Geometry: final body of the model. Coordinates: model frame, mm. Face numbers are marked on the shaded views. A direction names the side the tool comes from. Give positions to 0.01 mm unless a question says otherwise; leave off trailing zeros. Order: outer loops, then holes, each group sorted by start corner. A loop starts at its lowest first (then second) coordinate and runs counter-clockwise, first axis right, second up. Notation, with made-up numbers: M 4,8 L 62,8 A20 cw 62,16 Z; hole C 5,82 d10. An arc over 180 degrees is marked long. Use CSV: the item, a comma, the result in double quotes.
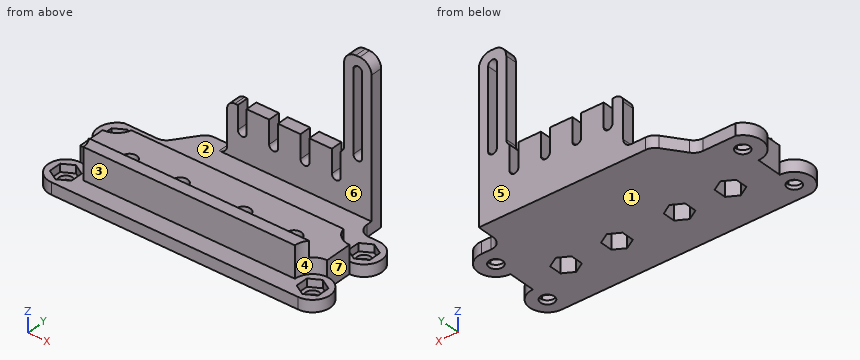
```python
from build123d import *

# Parameters (mm, degrees)
ESQUISSE1_R             = 1.749999998
BOSS_EXTRU_1_DEPTH      = 3
ENL_V_MAT_EXTRU_1_DEPTH = 2
ESQUISSE3_W             = 63
ESQUISSE3_H             = 15
BOSS_EXTRU_2_DEPTH      = 4
ESQUISSE5_W             = 63
ESQUISSE5_H             = 3
BOSS_EXTRU_3_DEPTH      = 4
ESQUISSE4_R             = 4.499999998
ESQUISSE4_R_2           = 4.527692567
ENL_V_MAT_EXTRU_2_DEPTH = 41.723100164
ESQUISSE6_R             = 1.875
ENL_V_MAT_EXTRU_4_DEPTH = 41.538511158
ENL_V_MAT_EXTRU_5_DEPTH = 4
ESQUISSE8_W             = 36.859122618
ESQUISSE8_H             = 3
BOSS_EXTRU_4_DEPTH      = 13
CONG_1_R                = 3
ESQUISSE9_W             = 7
ESQUISSE9_H             = 3
BOSS_EXTRU_5_DEPTH      = 25
CONG_2_R                = 3
CONG_3_R                = 2
CONG_4_R                = 2
ENL_V_MAT_EXTRU_6_DEPTH = 63.211313789


with BuildPart() as part:
    # Esquisse1 → Boss.-Extru.1 (new body)
    with BuildSketch(Plane.XY):
        with BuildLine():
            Line((-33.132757167, 9.120273973), (-23.272060479, 9.120273973))
            Line((-23.272060479, 9.120273973), (-17.824378499, 16.590273973))
            Line((-17.824378499, 16.590273973), (26.292187613, 16.590273973))
            Line((26.292187613, 16.590273973), (26.292187613, 9.120273973))
            Line((26.292187613, 9.120273973), (31.792187613, 9.120273973))
            ThreePointArc((31.792187613, 9.120273973), (36.319880182, 4.592581404), (31.792187613, 0.064888835))
            Line((31.792187613, 0.064888835), (31.792187613, -6.907418596))
            ThreePointArc((31.792187613, -6.907418596), (36.292187613, -11.407418596), (31.792187613, -15.907418596))
            Line((31.792187613, -15.907418596), (-31.207812389, -15.907418596))
            ThreePointArc((-31.207812389, -15.907418596), (-35.707812387, -11.407418595), (-31.207812387, -6.907418596))
            Line((-31.207812387, -6.907418596), (-31.207812387, -0.327318229))
            ThreePointArc((-31.207812387, -0.327318229), (-36.028663215, 3.610334136), (-33.132757167, 9.120273973))
        make_face()
        with Locations((-31.207812387, 4.592581404)):
            Circle(ESQUISSE1_R, mode=Mode.SUBTRACT)
        with Locations((-31.207812387, -11.407418596)):
            Circle(ESQUISSE1_R, mode=Mode.SUBTRACT)
        with Locations((31.792187613, 4.592581404)):
            Circle(ESQUISSE1_R, mode=Mode.SUBTRACT)
        with Locations((31.792187613, -11.407418596)):
            Circle(ESQUISSE1_R, mode=Mode.SUBTRACT)
    extrude(amount=BOSS_EXTRU_1_DEPTH)

    # Esquisse2 → Enlèv. mat.-Extru.1 (cut)
    with BuildSketch(Plane.XY.offset(3)):
        Polygon((-28.457812387, 6.180294644), (-31.207812387, 7.768007885), (-33.957812387, 6.180294644), (-33.957812387, 3.004868164), (-31.207812387, 1.417154924), (-28.457812387, 3.004868164), align=None)
        Polygon((-28.457812387, -9.819705356), (-31.207812387, -8.231992115), (-33.957812387, -9.819705356), (-33.957812387, -12.995131836), (-31.207812387, -14.582845076), (-28.457812387, -12.995131836), align=None)
        Polygon((29.042187613, -9.819705356), (29.042187613, -12.995131836), (31.792187613, -14.582845076), (34.542187613, -12.995131836), (34.542187613, -9.819705356), (31.792187613, -8.231992115), align=None)
        Polygon((29.042187613, 3.004868164), (31.792187613, 1.417154924), (34.542187613, 3.004868164), (34.542187613, 6.180294644), (31.792187613, 7.768007885), (29.042187613, 6.180294644), align=None)
    extrude(amount=-ENL_V_MAT_EXTRU_1_DEPTH, mode=Mode.SUBTRACT)

    # Esquisse3 → Boss.-Extru.2 (add)
    with BuildSketch(Plane.XY.offset(3)):
        with Locations((0.292187613, -3.907418596)):
            Rectangle(ESQUISSE3_W, ESQUISSE3_H)
    extrude(amount=BOSS_EXTRU_2_DEPTH)

    # Esquisse5 → Boss.-Extru.3 (add)
    with BuildSketch(Plane.XY.offset(7)):
        with Locations((0.292187613, -9.907418596)):
            Rectangle(ESQUISSE5_W, ESQUISSE5_H)
    extrude(amount=BOSS_EXTRU_3_DEPTH)

    # Esquisse4 → Enlèv. mat.-Extru.2 (cut, through all)
    with BuildSketch(Plane.XY.offset(3)):
        with Locations((-31.207812387, -11.407418596)):
            Circle(ESQUISSE4_R)
        with Locations((31.792187613, -11.407418596)):
            Circle(ESQUISSE4_R)
        with Locations((-31.207812387, 4.592581404)):
            Circle(ESQUISSE4_R_2)
        with Locations((31.792187613, 4.592581404)):
            Circle(ESQUISSE4_R_2)
    extrude(amount=ENL_V_MAT_EXTRU_2_DEPTH, mode=Mode.SUBTRACT)

    # Esquisse6 → Enlèv. mat.-Extru.4 (cut, through all)
    with BuildSketch(Plane.XY.offset(7)):
        with Locations((-20.707812387, -4.407418596)):
            Circle(ESQUISSE6_R)
        with Locations((-7.707812387, -4.407418596)):
            Circle(ESQUISSE6_R)
    enl_v_mat_extru_4 = extrude(amount=-ENL_V_MAT_EXTRU_4_DEPTH, mode=Mode.SUBTRACT)

    # Esquisse7 → Enlèv. mat.-Extru.5 (cut)
    with BuildSketch(Plane(origin=(0, 0, 0), x_dir=(-1, 0, 0), z_dir=(0, 0, -1))):
        Polygon((23.457812387, -2.819705356), (20.707812387, -1.231992115), (17.957812387, -2.819705356), (17.957812387, -5.995131836), (20.707812387, -7.582845076), (23.457812387, -5.995131836), align=None)
        Polygon((10.457812387, -2.819705356), (7.707812387, -1.231992115), (4.957812387, -2.819705356), (4.957812387, -5.995131836), (7.707812387, -7.582845076), (10.457812387, -5.995131836), align=None)
    enl_v_mat_extru_5 = extrude(amount=-ENL_V_MAT_EXTRU_5_DEPTH, mode=Mode.SUBTRACT)

    # Symétrie1: Enlèv. mat.-Extru.4, Enlèv. mat.-Extru.5 across plane
    add(enl_v_mat_extru_4.mirror(Plane(origin=(0.292187613, 0, 0), x_dir=(0, 0, 1), z_dir=(1, 0, 0))), mode=Mode.SUBTRACT)
    add(enl_v_mat_extru_5.mirror(Plane(origin=(0.292187613, 0, 0), x_dir=(0, 0, 1), z_dir=(1, 0, 0))), mode=Mode.SUBTRACT)

    # Esquisse8 → Boss.-Extru.4 (add)
    with BuildSketch(Plane.XY.offset(3)):
        with Locations((7.862626304, 15.090273973)):
            Rectangle(ESQUISSE8_W, ESQUISSE8_H)
    extrude(amount=BOSS_EXTRU_4_DEPTH)

    # Congé1
    cong_1_edges = [part.edges().sort_by_distance(p)[0] for p in [
        (-23.272060479, 9.120273973, 1.5),
        (-17.824378499, 16.590273973, 1.5),
        (26.292187613, 9.120273973, 1.5),
    ]]
    fillet(cong_1_edges, radius=CONG_1_R)

    # Esquisse9 → Boss.-Extru.5 (add)
    with BuildSketch(Plane.XY.offset(16)):
        with Locations((22.792187613, 15.090273973)):
            Rectangle(ESQUISSE9_W, ESQUISSE9_H)
    extrude(amount=BOSS_EXTRU_5_DEPTH)

    # Congé2
    cong_2_edges = [part.edges().sort_by_distance(p)[0] for p in [
        (19.292187613, 15.090273973, 41),
        (26.292187613, 15.090273973, 41),
    ]]
    fillet(cong_2_edges, radius=CONG_2_R)

    # Congé3
    cong_3_edges = [part.edges().sort_by_distance(p)[0] for p in [
        (19.292187613, 15.090273973, 16),
    ]]
    fillet(cong_3_edges, radius=CONG_3_R)

    # Congé4
    cong_4_edges = [part.edges().sort_by_distance(p)[0] for p in [
        (-10.566935005, 15.090273973, 3),
        (-10.566935005, 15.090273973, 16),
    ]]
    fillet(cong_4_edges, radius=CONG_4_R)

    # Esquisse10 → Enlèv. mat.-Extru.6 (cut, through all)
    with BuildSketch(Plane.XZ.offset(-13.590273973)):
        with BuildLine():
            Line((23.917187613, 37.5), (23.917187613, 17.088453941))
            ThreePointArc((23.917187613, 17.088453941), (22.792187613, 15.963453941), (21.667187613, 17.088453941))
            Line((21.667187613, 17.088453941), (21.667187613, 37.5))
            ThreePointArc((21.667187613, 37.5), (22.792187613, 38.625), (23.917187613, 37.5))
        make_face()
        with BuildLine():
            Line((18.417187613, 23.212933961), (18.417187613, 10.058154515))
            ThreePointArc((18.417187613, 10.058154515), (17.292187613, 8.933154515), (16.167187613, 10.058154515))
            Line((16.167187613, 10.058154515), (16.167187613, 23.212933961))
            ThreePointArc((16.167187613, 23.212933961), (17.292187613, 24.337933961), (18.417187613, 23.212933961))
        make_face()
        with BuildLine():
            Line((10.417187613, 23.212933961), (10.417187613, 10.058154515))
            ThreePointArc((10.417187613, 10.058154515), (9.292187613, 8.933154515), (8.167187613, 10.058154515))
            Line((8.167187613, 10.058154515), (8.167187613, 23.212933961))
            ThreePointArc((8.167187613, 23.212933961), (9.292187613, 24.337933961), (10.417187613, 23.212933961))
        make_face()
        with BuildLine():
            Line((2.417187613, 23.212933961), (2.417187613, 10.058154515))
            ThreePointArc((2.417187613, 10.058154515), (1.292187613, 8.933154515), (0.167187613, 10.058154515))
            Line((0.167187613, 10.058154515), (0.167187613, 23.212933961))
            ThreePointArc((0.167187613, 23.212933961), (1.292187613, 24.337933961), (2.417187613, 23.212933961))
        make_face()
        with BuildLine():
            Line((-5.582812387, 23.212933961), (-5.582812387, 10.058154515))
            ThreePointArc((-5.582812387, 10.058154515), (-6.707812387, 8.933154515), (-7.832812387, 10.058154515))
            Line((-7.832812387, 10.058154515), (-7.832812387, 23.212933961))
            ThreePointArc((-7.832812387, 23.212933961), (-6.707812387, 24.337933961), (-5.582812387, 23.212933961))
        make_face()
    extrude(amount=-ENL_V_MAT_EXTRU_6_DEPTH, mode=Mode.SUBTRACT)


solid = part.part
```
1. Reachability of the marked faces 4, 5, 6 and 7 from +Z, -Z, +X, -X, +Y, -Y: full face, straight path, thin tool, end or side. Return the list, or none.
Answer:
face 4,"+Z, +X, -Y"
face 5,"+Z, -Z, +X, -X, +Y"
face 6,"+Z, +X, -X"
face 7,"+Z, -Z, +X"
2. Line query: line 1 (Y direction, x = -29.5, z = 2); line 2 (Z direction, x = 21.5, y = 2.5); line 3 (Z direction, x = 15, y = 6.5). Output: solid intervals per line, ascending.
Answer:
line 1,"-15.91 to -13.6, -9.22 to 2.4, 6.78 to 9.12"
line 2,"0 to 7"
line 3,"0 to 3"
3. Section B-B, the plane x = 13.5. Return the cut outline in (y, z).
Answer:
outline,"M -15.91,0 L 16.59,0 L 16.59,16 L 13.59,16 L 13.59,3 L 3.59,3 L 3.59,7 L -8.41,7 L -8.41,11 L -11.41,11 L -11.41,3 L -15.91,3 Z"
4. Pull-direction query (Y, two-part tool) for the marked faces 1, 2 and 3; classes: +Y half, -Y half, draft (parallel to the pull), parting line (faces both ways), or undercut.
Answer:
face 1,"draft"
face 2,"undercut"
face 3,"-Y half"
5. Section A-A, the plane z = 28. Return the cut outline in (x, y), plus the area to 4 significant figures.
Answer:
outline,"M 19.29,13.59 L 21.67,13.59 L 21.67,16.59 L 19.29,16.59 Z; M 23.92,13.59 L 26.29,13.59 L 26.29,16.59 L 23.92,16.59 Z"
area,"14.25 mm2"
6. Pin query (flat end, axial travel): pin 1 Ø0.9 at (y, z) = (15.5, 11.5) entering from +X; pin 2 Ø4.5 at (x, y) = (33, -10.5) entering from +Z; pin 3 Ø10 at (y, z) = (8, 31.5) entering from +X; pin 4 Ø8 at (x, y) = (-14.5, -6) entering from +Z. Return the tip coordinate at first contact, or that it passes through.
Answer:
pin 1,"x = 26.29"
pin 2,"z = 3"
pin 3,"through"
pin 4,"z = 11"
7. Section C-C, the plane x = 25.5. Return the cut outline in (y, z).
Answer:
outline,"M -15.91,0 L 16.59,0 L 16.59,40.03 L 13.59,40.03 L 13.59,3 L 3.59,3 L 3.59,7 L -8.41,7 L -8.41,11 L -11.41,11 L -11.41,3 L -15.91,3 Z"
